The listing builds one solid part. Answer for the finished solid, in the listing's coordinates (mm). Give positions to 0.01 mm unless a question says otherwise; leave off trailing zeros. Write each loop counter-clockwise with the first axis right and the second up, starting at its lowest first coordinate (ties: lowest second). Pieces come first, ordered by that corner, then holes. Notation, with made-up numbers: (75, 65.25) - (107, 65.25) arc R21 ccw to (107, 98.25) - close; hole circle Ø9 at (18, -11). An arc over 180 degrees is marked (long way). One line per question, with ' | ' between items. Start each with the question number.
1. The mould has two halves that part along Y. Classify faces 1 (the face through (-38, 65, 3.175)), 2 (the face through (-28, 0, 2)), 3 (the face through (-5.724, 74.198, 1.61)): +Y half, -Y half, draft (parallel to the pull), parting line (faces both ways), or undercut.
2. A cutting plane is placed at B-B (x = -22). Determine the outline of the cut face in (y, z) (3 decimals), then the cut area to 3 significant figures.
3. A cutting plane is placed at A-A (y = 44.45). Determine the outline of the cut face in (x, z) (3 decimals).
4. Find the intervals of material crossed by L1, parallel to Y at x = -47.5, z = 0.95; L2, parallel to X at y = 43.5, z = 3.05; L3, parallel to Y at x = -60, z = 0.3, in increasing order. Write a range as from..to.
5. A cutting plane is placed at C-C (z = 1.9). State how many separate pieces and enclosed holes the cut face has, then the cut area to 3 significant figures.
Autodesk Inventor part; units mm, degrees
ref_plane "YZ Plane" through (0, 0, 0) normal (1, 0, 0) x (0, 1, 0)
ref_plane "XZ Plane" through (0, 0, 0) normal (0, 1, 0) x (-1, 0, 0)
ref_plane "XY Plane" through (0, 0, 0) normal (0, 0, 1) x (1, 0, 0)
sketch "Sketch1" plane through (0, 0, 0) normal (0, 0, 1) x (1, 0, 0)
  line L0 (0, 0) -> (-56.9976, 0)
  line L1 (-56.9976, 88.9) -> (0, 88.9)
  line L2 (0, 88.9) -> (-7.493, 88.9)
  line L3 (-7.493, 88.9) -> (-7.493, 82.55)
  line L4 (-56.9976, 88.9) -> (-49.5046, 88.9)
  line L5 (-49.5046, 88.9) -> (-49.5046, 82.55)
  line L6 (-56.9976, 88.9) -> (-69.6976, 88.9)
  line L7 (-69.6976, 88.9) -> (-69.6976, 0)
  line L8 (-69.6976, 0) -> (-56.9976, 0)
  line L9 (0, 88.9) -> (8.89, 88.9)
  line L10 (8.89, 0) -> (0, 0)
  line L11 (0, 88.9) -> (12.7, 88.9)
  line L12 (12.7, 88.9) -> (12.7, 0)
  line L13 (12.7, 0) -> (0, 0)
  dimension "d1" = 56.9976
  dimension "d2" = 88.9
  dimension "d3" = 7.493
  dimension "d4" = 6.35
  dimension "d5" = 7.493
  dimension "d19" = 6.35
  dimension "d48" = 12.7
  dimension "d57" = 12.7
extrude "Plate5" add sketch "Sketch1" along normal blind 3.175
sketch "Sketch7" plane through (12.7, 0, 0) normal (1, 0, 0) x (0, 0, -1)
  line L0 (-3.175, 88.9) -> (-3.175, 0)
  line L1 (0, 0) -> (-3.175, 0)
  line L2 (0, 0) -> (0, 88.9)
  line L3 (0, 88.9) -> (-3.175, 88.9)
sketch "Sketch11" plane through (0, 0, 3.175) normal (0, 0, 1) x (1, 0, 0)
  circle A0 centre (-7.4976, 71.4155) radius 3.3
  circle A1 centre (-49.4976, 71.4155) radius 3.3
  circle A2 centre (5.484, 10.4813) radius 3.2
  line L0 (-11.9976, 581.6155) -> (-11.9976, -78.7845)
  circle A3 centre (5.484, 10.4813) radius 3.2
  line L1 (-53.516, -9.5187) -> (-68.516, -9.5187)
  line L2 (-68.516, 30.4813) -> (-68.516, -9.5187)
  line L3 (-68.516, 30.4813) -> (-53.516, 30.4813)
  line L4 (-53.516, 30.4813) -> (-53.516, -9.5187)
  circle A4 centre (-62.516, 10.4813) radius 3.2
  circle A5 centre (-62.516, 10.4813) radius 3.2
  point P0 (0, 0)
  point P1 (-28.516, 7.2815)
extrude "Cut5" cut sketch "Sketch11" against normal blind 3.175 contours A0 | A1 | A2 | A4
sketch "Sketch12" plane through (0, 0, 3.175) normal (0, 0, 1) x (1, 0, 0)
  line L0 (-69.6976, 88.9) -> (12.7, 88.9)
  line L1 (-69.6976, 0) -> (-69.6976, 88.9)
  line L2 (-28.4988, 88.9) -> (-28.4988, 44.45)
  circle A0 centre (-28.4988, 44.45) radius 22.225
  point P0 (0, 0)
  dimension "d71" = 44.45
extrude "Cut6" cut sketch "Sketch12" against normal blind 3.175
equation "\"d69\" = Thickness"
equation "\"d72\" = Thickness"
equation "\"BendRadius\" = Thickness"
equation "\"BendReliefWidth\" = Thickness"
equation "\"BendReliefDepth\" = 0.5 * Thickness"
equation "\"CornerReliefSize\" = 4 * Thickness"
equation "\"MinimumRemnant\" = 2 * Thickness"
equation "\"TransitionRadius\" = BendRadius"
equation "\"JacobiRadiusSize\" = BendRadius"
equation "\"GapSize\" = Thickness"
equation "\"d8\" = BendRadius"
equation "\"d56\" = BendRadius"
properties part number "upper face mount" material "Aluminum 6061"
Determined:
1) face 1: draft | face 2: -Y half | face 3: undercut
2) outline: (0, 0) - (23.196, 0) - (23.196, 3.175) - (0, 3.175) - close; (65.704, 0) - (88.9, 0) - (88.9, 3.175) - (65.704, 3.175) - close | area: 147 mm2
3) outline: (-69.698, 0) - (-50.724, 0) - (-50.724, 3.175) - (-69.698, 3.175) - close; (-6.274, 0) - (12.7, 0) - (12.7, 3.175) - (-6.274, 3.175) - close
4) L1: 0..32.92, 55.98..68.79, 74.04..88.9 | L2: -69.7..-50.7, -6.29..12.7 | L3: 0..8.5, 12.46..88.9
5) separate pieces: 1 | enclosed holes: 5 | area: 5,640 mm2
